```python
from build123d import *

# Parameters (mm, degrees)
F0_W     = 88.9
F0_H     = 165.1
F1_DEPTH = 6.35
F2_DEPTH = 25.4
F3_DEPTH = 50.8
F4_R     = 6.34999
F5_SIZE2 = 12.7
F5_SIZE  = 7.3323484187
F6_SIZE2 = 12.7
F6_SIZE  = 7.3323484187
F7_SIZE2 = 12.7
F7_SIZE  = 7.3323484187


# Not quite as in the source:
# - a fillet or chamfer is up to 0.001 mm smaller than in the source, because OpenCascade refuses the exact size


with BuildPart() as f1:
    # F0 (on Top) → F1 (new body)
    with BuildSketch(Plane.XY):
        with Locations((-38.1, 76.2)):
            Rectangle(F0_W, F0_H)
        Polygon((-76.2, 114.3), (-76.2, 152.4), (-38.1, 152.4), (0, 152.4), (0, 38.1), (0, 0), (-38.1, 0), (-76.2, 0), align=None, mode=Mode.SUBTRACT)
    extrude(amount=F1_DEPTH)

    # F0 (on Top) → F2 (join)
    with BuildSketch(Plane.XY):
        with BuildLine():
            Line((0, 152.4), (-38.1, 152.4))
            Line((-38.1, 152.4), (-38.1, 127))
            ThreePointArc((-38.1, 127), (-41.8197438789, 118.0197438789), (-50.8, 114.3))
            Line((-50.8, 114.3), (-76.2, 114.3))
            Line((-76.2, 114.3), (-76.2, 0))
            Line((-76.2, 0), (-38.1, 0))
            Line((-38.1, 0), (-38.1, 25.4))
            ThreePointArc((-38.1, 25.4), (-34.3802561211, 34.3802561211), (-25.4, 38.1))
            Line((-25.4, 38.1), (0, 38.1))
            Line((0, 38.1), (0, 152.4))
        make_face()
    extrude(amount=F2_DEPTH)

    # F0 (on Top) → F3 (join)
    with BuildSketch(Plane.XY):
        with BuildLine():
            Line((-38.1, 152.4), (-76.2, 152.4))
            Line((-76.2, 152.4), (-76.2, 114.3))
            Line((-76.2, 114.3), (-50.8, 114.3))
            ThreePointArc((-50.8, 114.3), (-41.8197438789, 118.0197438789), (-38.1, 127))
            Line((-38.1, 127), (-38.1, 152.4))
        make_face()
        with BuildLine():
            Line((0, 0), (0, 38.1))
            Line((0, 38.1), (-25.4, 38.1))
            ThreePointArc((-25.4, 38.1), (-34.3802561211, 34.3802561211), (-38.1, 25.4))
            Line((-38.1, 25.4), (-38.1, 0))
            Line((-38.1, 0), (0, 0))
        make_face()
    extrude(amount=F3_DEPTH)

    # F4 (radius 6.35 in the source; OpenCascade refuses exactly that, so slightly less here)
    f4_edges = [f1.edges().sort_by_distance(p)[0] for p in [
        (6.35, 76.2, 6.35),
        (-38.1, 158.75, 6.35),
        (-82.55, 76.2, 6.35),
        (-38.1, -6.35, 6.35),
    ]]
    fillet(f4_edges, radius=F4_R)

    # F5
    f5_edges = [f1.edges().sort_by_distance(p)[0] for p in [
        (0, 95.25, 25.4),
        (-57.15, 0, 25.4),
        (-76.2, 57.15, 25.4),
        (-19.05, 152.4, 25.4),
    ]]
    f5_side = f1.faces().sort_by_distance((-38.1, 76.2, 25.4))[0]
    chamfer(f5_edges, length=F5_SIZE, length2=F5_SIZE2, reference=f5_side)

    # F6
    f6_edges = [f1.edges().sort_by_distance(p)[0] for p in [
        (-57.15, 152.4, 50.8),
        (-76.2, 133.35, 50.8),
    ]]
    f6_side = f1.faces().sort_by_distance((-57.546042, 133.746042, 50.8))[0]
    chamfer(f6_edges, length=F6_SIZE, length2=F6_SIZE2, reference=f6_side)

    # F7
    f7_edges = [f1.edges().sort_by_distance(p)[0] for p in [
        (0, 19.05, 50.8),
        (-19.05, 0, 50.8),
    ]]
    f7_side = f1.faces().sort_by_distance((-18.653958, 18.653958, 50.8))[0]
    chamfer(f7_edges, length=F7_SIZE, length2=F7_SIZE2, reference=f7_side)


solid = f1.part
```
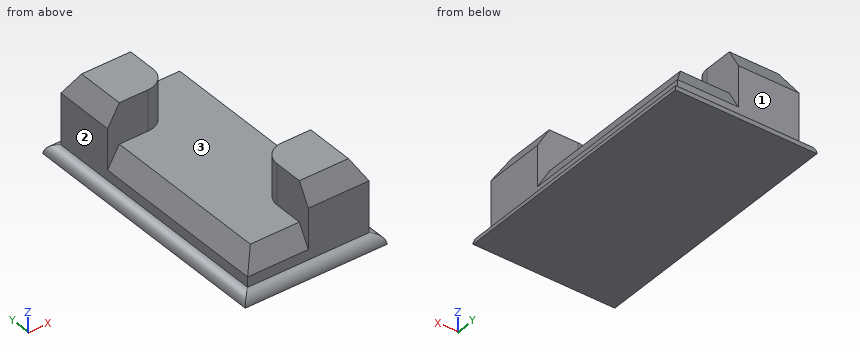
Here's how the part is built. I have some questions about the finished solid (model axes, mm). Face numbers are marked on the shaded views. A direction names the side the tool comes from. Coordinates: 2 decimals unless noted, no trailing zeros. Loops run counter-clockwise (first coordinate to the right, second up) from the corner with the lowest first, then second, coordinate; pieces in that order, holes last. Notation, with made-up numbers: (0.5, -14.75) - (36.5, -14.75) arc R29 cw to (36.5, 17.25) - close; hole circle Ø6 at (10.25, -17.5). An arc over 180 degrees is marked (long way). Return JSON: item names as keys, results as strings. Group by question number.
Item 1: If we section it at C-C on z = 22: Write out the boundary of the cut face in (x, y).
Item 2: On a 3-axis mill with a long thin cutter (end or side, diameter ignored), from which of +Z, -Z, +X, -X, +Y, -Y can I reach the whole of each face in a straight line? I mean the marked faces 1, 2 and 3. Say none if no direction works.
Item 3: I need wall thicknesses on line 1 (X direction, y = 38, z = 10); line 2 (Z direction, x = -44, y = 25.5); line 3 (X direction, y = 145.5, z = 26). Which ranges of each line are inside material? Lowest first, please. Write a range as from..to.
Item 4: Will these pins go through, and if not, where does the flat tip stop? P1, Ø6, axis at y = 137.5, z = 40.5, coming from the +X side; P2, Ø5, axis at x = -60, z = 19.5, coming from the -Y side; P3, Ø1, axis at x = -23, z = 39.5, coming from the +Y side.
Calculated:
{
 "1": {"outline": "(-76.2, 114.3) - (-70.83, 114.3) - (-70.83, 5.37) - (-38.1, 5.37) - (-38.1, 0) - (0, 0) - (0, 38.1) - (-5.37, 38.1) - (-5.37, 147.03) - (-38.1, 147.03) - (-38.1, 152.4) - (-76.2, 152.4) - close"},
 "2": {"face 1": "+Z, +X, -X, +Y", "face 2": "+Z, -X, +Y, -Y", "face 3": "+Z"},
 "3": {"line 1": "x = -76.2..0", "line 2": "z = 0..25.4", "line 3": "x = -76.2..-38.1"},
 "4": {"P1": "stops at x = -38.1", "P2": "stops at y = 2.48", "P3": "stops at y = 38.1"}
}
